Autodesk Inventor part; units mm, degrees
ref_plane "YZ Plane" through (0, 0, 0) normal (1, 0, 0) x (0, 1, 0)
ref_plane "XZ Plane" through (0, 0, 0) normal (0, 1, 0) x (-1, 0, 0)
ref_plane "XY Plane" through (0, 0, 0) normal (0, 0, 1) x (1, 0, 0)
sketch "Sketch1" plane through (0, 0, 0) normal (0, 0, 1) x (1, 0, 0)
  circle A0 centre (0, 0) radius 14.2875
  circle A1 centre (0, 0) radius 20.32 construction
  circle A2 centre (0, 50.8) radius 30.48 construction
  circle A3 centre (0, 50.8) radius 14.2875
  circle A4 centre (0, 50.8) radius 35.56 construction
  circle A5 centre (0, 0) radius 25.4 construction
  line L0 (34.8415, 43.688) -> (24.8868, -5.08)
  line L1 (-34.8415, 43.688) -> (-24.8868, -5.08)
  arc A6 (34.8415, 43.688) -> (-34.8415, 43.688) centre (0, 50.8) ccw
  arc A7 (-24.8868, -5.08) -> (24.8868, -5.08) centre (0, 0) ccw
  dimension "d0" = 28.575
  dimension "d2" = 40.64
  dimension "d6" = 60.96
  dimension "d7" = 28.575
  dimension "d9" = 5.08
  dimension "d10" = 5.08
extrude "Extrusion1" add sketch "Sketch1" along normal mid plane 6.35
properties part number "Revised Gearbox Plate #1" material "Aluminum 6061"
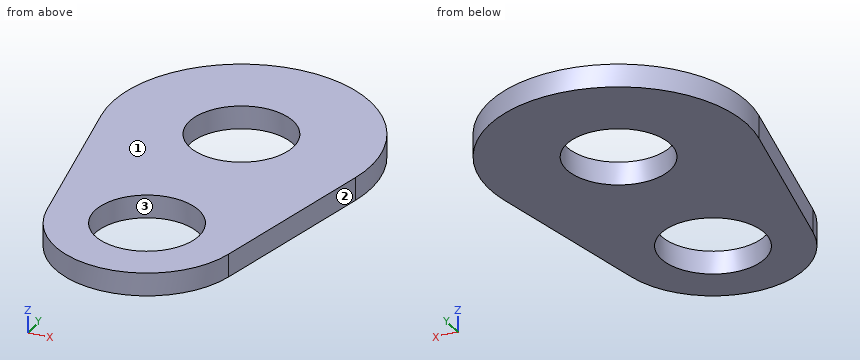
CAD build for the part. Positions are in the model's coordinates, mm. Face numbers are marked on the shaded views. Round coordinates to 2 decimals unless told otherwise and drop trailing zeros. Write each loop counter-clockwise with the first axis right and the second up, starting at its lowest first coordinate (ties: lowest second). Pieces come first, ordered by that corner, then holes. Notation, with made-up numbers: (-18.75, 48) - (16.25, 48) arc R27 ccw to (16.25, 82) - close; hole circle Ø8 at (66, 13). An arc over 180 degrees is marked (long way). Write item = value, one per line. Start each with the question number.
Q1. Band-saw the part on B-B (y = 50.8). Give the cut face in (x, z) (1 decimal), then the cut area to 3 significant figures.
Q2. Mould opens along Y. For the marked faces 1, 2 and 3 say: pulls with the +Y half, pulls with the -Y half, needs draft (parallel to the pull), parting line crosses it, or undercut.
Q3. Band-saw the part on D-D (x = 8.5). Give the cut face in (y, z) (3 decimals), then the cut area to 3 significant figures.
Q4. Band-saw the part on C-C (z = 0.25). Give the cut face in (x, y) (1 decimal).
Q5. Probe L1, parallel to Y at x = -3, z = -2.25; L2, parallel to Y at x = 12.5, z = 1; L3, parallel to X at y = -3.5, z = -1. List the from-to ranges inside material, lowest first. Write a range as from..to.
Q6. Drop flat-ended pins along their axis: pin 1 (3 mm diameter, centred on y = 20.5, z = 0.5, fed in from -X); pin 2 (1 mm diameter, centred on x = 2.5, z = -2, fed in from -Y); pin 3 (2 mm diameter, centred on y = 70, z = 0, fed in from +X). Give the stop position or say it passes through.
Q7. Band-saw the part on A-A (x = 0). Give the cut face in (y, z) (1 decimal).
Answers below:
q1.outline = (-35.6, -3.2) - (-14.3, -3.2) - (-14.3, 3.2) - (-35.6, 3.2) - close; (14.3, -3.2) - (35.6, -3.2) - (35.6, 3.2) - (14.3, 3.2) - close
q1.area = 270 mm2
q2.face_1 = needs draft
q2.face_2 = pulls with the -Y half
q2.face_3 = undercut
q3.outline = (-23.936, -3.175) - (-11.484, -3.175) - (-11.484, 3.175) - (-23.936, 3.175) - close; (11.484, -3.175) - (39.316, -3.175) - (39.316, 3.175) - (11.484, 3.175) - close; (62.284, -3.175) - (85.329, -3.175) - (85.329, 3.175) - (62.284, 3.175) - close
q3.area = 402 mm2
q4.outline = (-34.8, 43.7) - (-24.9, -5.1) arc R25.4 ccw to (24.9, -5.1) - (34.8, 43.7) arc R35.6 ccw (long way) to start; hole circle Ø28.6 at (0, 0); hole circle Ø28.6 at (0, 50.8)
q5.L1 = -25.22..-13.97, 13.97..36.83, 64.77..86.23
q5.L2 = -22.11..-6.92, 6.92..43.88, 57.72..84.09
q5.L3 = -25.21..-13.85, 13.85..25.21
q6.pin_1 = -30.41
q6.pin_2 = -25.32
q6.pin_3 = 30.55
q7.outline = (-25.4, -3.2) - (-14.3, -3.2) - (-14.3, 3.2) - (-25.4, 3.2) - close; (14.3, -3.2) - (36.5, -3.2) - (36.5, 3.2) - (14.3, 3.2) - close; (65.1, -3.2) - (86.4, -3.2) - (86.4, 3.2) - (65.1, 3.2) - close
